from build123d import *

# Parameters (mm, degrees)
SKETCH2_R           = 2.778125
BOSS_EXTRUDE2_DEPTH = 56.3835756
SKETCH3_R           = 1.651
CUT_EXTRUDE1_DEPTH  = 23.5668
SKETCH4_W           = 10.767766953
SKETCH4_H           = 3
CUT_EXTRUDE2_DEPTH  = 3.75
SKETCH5_R           = 2.8
CUT_EXTRUDE3_DEPTH  = 80.995318373
CUT_EXTRUDE4_DEPTH  = 77.107177875
CUT_EXTRUDE5_DEPTH  = 4


with BuildPart() as part:
    # Sketch2 → Boss-Extrude2 (new body)
    with BuildSketch(Plane(origin=(0, 0, 0), x_dir=(0, 0, -1), z_dir=(1, 0, 0))):
        with BuildLine():
            Line((0, 25.778125), (30, 25.778125))
            ThreePointArc((30, 25.778125), (31.964431026, 24.964431026), (32.778125, 23))
            Line((32.778125, 23), (32.778125, 14.278125))
            ThreePointArc((32.778125, 14.278125), (31.964431026, 12.313693974), (30, 11.5))
            Line((30, 11.5), (30, 6.906829453))
            Line((30, 6.906829453), (31.767766953, 5.1390625))
            Line((31.767766953, 5.1390625), (46.767766953, 5.1390625))
            Line((46.767766953, 5.1390625), (46.767766953, 32.1390625))
            Line((46.767766953, 32.1390625), (-16.767766953, 32.1390625))
            Line((-16.767766953, 32.1390625), (-16.767766953, 5.1390625))
            Line((-16.767766953, 5.1390625), (-1.767766953, 5.1390625))
            Line((-1.767766953, 5.1390625), (0, 6.906829453))
            Line((0, 6.906829453), (0, 11.5))
            ThreePointArc((0, 11.5), (-1.964431026, 12.313693974), (-2.778125, 14.278125))
            Line((-2.778125, 14.278125), (-2.778125, 23))
            ThreePointArc((-2.778125, 23), (-1.964431026, 24.964431026), (0, 25.778125))
        make_face()
        with Locations((-10, 26.6390625)):
            Circle(SKETCH2_R, mode=Mode.SUBTRACT)
        with Locations((-10, 10.6390625)):
            Circle(SKETCH2_R, mode=Mode.SUBTRACT)
        with Locations(Location((40, 10.6390625, 0), (0, 0, 180))):
            Circle(SKETCH2_R, mode=Mode.SUBTRACT)
        with Locations(Location((40, 26.6390625, 0), (0, 0, 180))):
            Circle(SKETCH2_R, mode=Mode.SUBTRACT)
    extrude(amount=BOSS_EXTRUDE2_DEPTH)

    # Sketch3 → Cut-Extrude1 (cut)
    with BuildSketch(Plane(origin=(56.3835756, 0, 0), x_dir=(0, 0, -1), z_dir=(1, 0, 0))):
        with Locations((-10, 18.6390625)):
            Circle(SKETCH3_R)
        with Locations(Location((40, 18.6390625, 0), (0, 0, 180))):
            Circle(SKETCH3_R)
    cut_extrude1 = extrude(amount=-CUT_EXTRUDE1_DEPTH, mode=Mode.SUBTRACT)

    # Sketch4 → Cut-Extrude2 (cut, symmetric)
    with BuildSketch(Plane(origin=(0, 18.6390625, 0), x_dir=(0, 0, -1), z_dir=(0, -1, 0))):
        with Locations((-11.383883477, 44.8835756)):
            Rectangle(SKETCH4_W, SKETCH4_H)
        with Locations((41.383883477, 44.8835756)):
            Rectangle(SKETCH4_W, SKETCH4_H)
        with Locations((-11.383883477, 8.5)):
            Rectangle(SKETCH4_W, SKETCH4_H)
        with Locations((41.383883477, 8.5)):
            Rectangle(SKETCH4_W, SKETCH4_H)
    extrude(amount=CUT_EXTRUDE2_DEPTH, both=True, mode=Mode.SUBTRACT)

    # Sketch5 → Cut-Extrude3 (cut, through all)
    with BuildSketch(Plane(origin=(56.3835756, 0, 0), x_dir=(0, 0, -1), z_dir=(1, 0, 0))):
        with Locations((-10, 26.6390625)):
            Circle(SKETCH5_R)
        with Locations((0, 23)):
            Circle(SKETCH5_R)
        with Locations((-10, 10.6390625)):
            Circle(SKETCH5_R)
        with Locations((40, 26.6390625)):
            Circle(SKETCH5_R)
        with Locations((40, 10.6390625)):
            Circle(SKETCH5_R)
        with Locations((30, 23)):
            Circle(SKETCH5_R)
        with Locations((0, 14.278125)):
            Circle(SKETCH5_R)
        with Locations((30, 14.278125)):
            Circle(SKETCH5_R)
    extrude(amount=-CUT_EXTRUDE3_DEPTH, mode=Mode.SUBTRACT)

    # Mirror1: Cut-Extrude1 across plane
    add(cut_extrude1.mirror(Plane.ZY.offset(-28.1917878)), mode=Mode.SUBTRACT)

    # Sketch6 → Cut-Extrude4 (cut, through all)
    with BuildSketch(Plane.XZ.offset(-25.778125)):
        with BuildLine():
            Line((11.737987423, -5), (10.250411309, -3.608694115))
            ThreePointArc((10.250411309, -3.608694115), (7.044145412, -5), (10.250411309, -6.391305885))
            Line((10.250411309, -6.391305885), (11.737987423, -5))
        make_face()
        with BuildLine():
            Line((50.223272198, -5), (48.735696084, -3.608694115))
            ThreePointArc((48.735696084, -3.608694115), (45.529430188, -5), (48.735696084, -6.391305885))
            Line((48.735696084, -6.391305885), (50.223272198, -5))
        make_face()
        with BuildLine():
            Line((50.223272198, -25), (48.735696084, -26.391305885))
            ThreePointArc((48.735696084, -26.391305885), (45.529430188, -25), (48.735696084, -23.608694115))
            Line((48.735696084, -23.608694115), (50.223272198, -25))
        make_face()
        with BuildLine():
            Line((11.737987423, -25), (10.250411309, -23.608694115))
            ThreePointArc((10.250411309, -23.608694115), (7.044145412, -25), (10.250411309, -26.391305885))
            Line((10.250411309, -26.391305885), (11.737987423, -25))
        make_face()
    extrude(amount=-CUT_EXTRUDE4_DEPTH, mode=Mode.SUBTRACT)

    # Sketch7 → Cut-Extrude5 (cut)
    with BuildSketch(Plane(origin=(0, 25.778125, 0), x_dir=(-1, 0, 0), z_dir=(0, -1, 0))):
        Polygon((-10.921547137, 28.4163), (-12.893948862, 25), (-10.921547137, 21.5837), (-6.976743688, 21.5837), (-5.004341963, 25), (-6.976743688, 28.4163), align=None)
        Polygon((-10.921547137, 8.4163), (-12.893948862, 5), (-10.921547137, 1.5837), (-6.976743688, 1.5837), (-5.004341963, 5), (-6.976743688, 8.4163), align=None)
        Polygon((-45.462028463, 8.4163), (-49.406831912, 8.4163), (-51.379233637, 5), (-49.406831912, 1.5837), (-45.462028463, 1.5837), (-43.489626738, 5), align=None)
        Polygon((-45.462028463, 28.4163), (-49.406831912, 28.4163), (-51.379233637, 25), (-49.406831912, 21.5837), (-45.462028463, 21.5837), (-43.489626738, 25), align=None)
    extrude(amount=-CUT_EXTRUDE5_DEPTH, mode=Mode.SUBTRACT)


solid = part.part
Model file for the job. Use its own axes, mm. A direction names the side the tool comes from. Round coordinates to 2 decimals unless told otherwise and drop trailing zeros. Order: outer loops, then holes, each group sorted by start corner. A loop starts at its lowest first (then second) coordinate and runs counter-clockwise, first axis right, second up.
(1) Band-saw the part on C-C (z = -40). Give the number of separate pieces and of enclosed holes in the cut face, then the cut area to 3 significant figures.
(2) 3-axis set-ups, long thin cutter, end or side, ignore diameter. For faces 4 (the face through (9, 28, -8.416)), 5 (the face through (28, 19, -32.778)), 6 (the face through (38.174, 18.143, -38.425)), 7 (the face through (11, 30.94, -24.31)): which of +Z, -Z, +X, -X, +Y, -Y reach the whole face in a straight line?
(3) Pin check, flat tips, straight feed: pin 1 (8 mm diameter, centred on y = 18, z = -39, fed in from +X); pin 2 (5 mm diameter, centred on y = 23, z = -6, fed in from -X); pin 3 (2 mm diameter, centred on y = 18.64, z = -40, fed in from +X); pin 4 (4.5 mm diameter, centred on x = 47.43, z = -5, fed in from -Y). Stop position of each tip, or through.
(4) Band-saw the part on A-A (y = 8.75). List the corners of the cut face in (x, z).
(5) Drill centre lines: line 1 (Y direction, x = 35.5, z = -40); line 2 (X direction, y = 22.25, z = -37); line 3 (Z direction, x = 46, y = 14.5). Where is each one in solid material? Low to high.
(6) Pull direction Y, two halves, no side cores. Call faces 1 (the face through (43.384, 19, 13)), 2 (the face through (46, 29.778, -27)), 3 (the face through (49.469, 30.942, -5.705)): released by +Y, released by -Y, zero draft, split by the parting line, or undercut.
(7) Band-saw the part on B-B (x = 14). List the corners of the cut face in (y, z).
Verdict:
1. separate pieces: 3
1. enclosed holes: 0
1. area: 710 mm2
2. face 4: -Y
2. face 5: +X, -X
2. face 6: +X
2. face 7: +Y, -Y
3. pin 1: stops at x = 56.38
3. pin 2: passes through
3. pin 3: stops at x = 32.82
3. pin 4: stops at y = 29.78
4. outline: (0, -46.77) - (56.38, -46.77) - (56.38, -42.07) - (0, -42.07) - close; (0, -37.93) - (56.38, -37.93) - (56.38, -30) - (0, -30) - close; (0, 0) - (56.38, 0) - (56.38, 7.93) - (0, 7.93) - close; (0, 12.07) - (56.38, 12.07) - (56.38, 16.77) - (0, 16.77) - close
5. line 1: y = 5.14 to 7.84, 13.44 to 16.99, 20.29 to 23.84, 29.44 to 32.14
5. line 2: x = 0 to 7, 10 to 43.38, 46.38 to 56.38
5. line 3: z = -46.77 to -32.79, 2.79 to 16.77
6. face 1: undercut
6. face 2: released by -Y
6. face 3: zero draft
7. outline: (5.14, -46.77) - (32.14, -46.77) - (32.14, 16.77) - (5.14, 16.77) - (5.14, 1.77) - (6.91, 0) - (11.48, 0) arc R2.8 cw to (14.63, 2.78) - (22.65, 2.78) arc R2.8 cw to (25.78, -0.35) - (25.78, -29.65) arc R2.8 cw to (22.65, -32.78) - (14.63, -32.78) arc R2.8 cw to (11.48, -30) - (6.91, -30) - (5.14, -31.77) - close; hole circle Ø5.6 at (10.64, -40); hole circle Ø5.6 at (10.64, 10); hole circle Ø3.3 at (18.64, -40); hole circle Ø3.3 at (18.64, 10); hole circle Ø5.6 at (26.64, -40); hole circle Ø5.6 at (26.64, 10)
